Read the model definition and answer for the solid it produces. Units are mm, in the model's axes. Give positions to 0.01 mm unless a question says otherwise; leave off trailing zeros. Write each loop counter-clockwise with the first axis right and the second up, starting at its lowest first coordinate (ties: lowest second). Pieces come first, ordered by that corner, then holes. Notation, with made-up numbers: M 22,35.25 L 50,35.25 A30 ccw 50,67.25 Z; hole C -14.75,76 d9. An arc over 180 degrees is marked long. Put each result on its own line as item: value.
from build123d import *

# Parameters (mm, degrees)
SKETCH_1_W               = 310
SKETCH_1_H               = 170
EXTRUDE_1_DEPTH          = 3
CUT_EXTRUDE_1_DEPTH      = 177.802149308
CUT_EXTRUDE_1_DEPTH_BACK = 177.802149308
CHAMFER_1_SIZE           = 45


with BuildPart() as part:
    # 草图1 → 凸台-拉伸1 (new body)
    with BuildSketch(Plane(origin=(0, 0, 0), x_dir=(1, 0, 0), z_dir=(0, 1, 0))):
        Rectangle(SKETCH_1_W, SKETCH_1_H)
    extrude(amount=EXTRUDE_1_DEPTH)

    # 草图2 → 切除-拉伸1 (cut, two sides: drawn at the far end of the back side and taken through both)
    with BuildSketch(Plane(origin=(0, 3, 0), x_dir=(1, 0, 0), z_dir=(0, 1, 0)).offset(-CUT_EXTRUDE_1_DEPTH_BACK)):
        Polygon((-20, -50), (-40, -85), (40, -85), (20, -50), align=None)
    extrude(amount=CUT_EXTRUDE_1_DEPTH + CUT_EXTRUDE_1_DEPTH_BACK, mode=Mode.SUBTRACT)

    # 倒角1
    chamfer_1_edges = [part.edges().sort_by_distance(p)[0] for p in [
        (-155, 1.5, -85),
        (155, 1.5, -85),
    ]]
    chamfer(chamfer_1_edges, length=CHAMFER_1_SIZE)


solid = part.part
(1) Section C-C on x = -7 is taken. Determine the outline of the cut face in (y, z).
Result:
outline: M 0,-85 L 3,-85 L 3,50 L 0,50 Z
(2) Section B-B on z = -47 is taken. Determine the outline of the cut face in (x, y).
Result:
outline: M -148,0 L 148,0 L 148,3 L -148,3 Z
(3) For a pull along X with two mould halves and no side action, classify faces 1 (the face through (-29.86, 1.479, 67.255)), 2 (the face through (-132, 1, -63)), 3 (the face through (30.14, 1.479, 67.745)), 4 (the face through (-2, 0, -1)) as +X half, -X half, draft (parallel to the pull), parting line (faces both ways), or undercut.
Result:
face 1: undercut
face 2: -X half
face 3: undercut
face 4: draft
(4) Straight lines are drawn through the part: line 1 along Z through (x, y) = (-20, 0.85); line 2 along X through (y, z) = (1.7, 75); line 3 along X through (y, z) = (2.9, -72.5). For each, find the intervals that lie inside material, in ascending order. Write a range as from..to.
Result:
line 1: z = -85..50
line 2: x = -155..-34.29, 34.29..155
line 3: x = -122.5..122.5
(5) Section A-A on y = 1.15 is taken. Determine the outline of the cut face in (x, z).
Result:
outline: M -155,-40 L -110,-85 L 110,-85 L 155,-40 L 155,85 L 40,85 L 20,50 L -20,50 L -40,85 L -155,85 Z
(6) Given pin 1 Ø12 at (x, z) = (34.5, 55.5) entering from -Y; pin 2 Ø1.5 at (x, y) = (7, 1) entering from +Z, each flat-ended and moving along its own axis, determine where each tip first touches the part or whether it passes through.
Result:
pin 1: stops at y = 0
pin 2: stops at z = 50
